Check sheet for the modelled part. Datum: model origin and axes. Units: mm. Face numbers are marked on the shaded views. Give positions to 0.01 mm unless a question says otherwise; leave off trailing zeros. Order: outer loops, then holes, each group sorted by start corner. A loop starts at its lowest first (then second) coordinate and runs counter-clockwise, first axis right, second up. Notation, with made-up numbers: (53, -22.75) -> (68, -22.75) arc R10 cw to (68, -13.75) -> close; hole circle Ø6 at (76, 40.25). An arc over 180 degrees is marked (long way). Write each question's results on one line, items separated by ' | '.
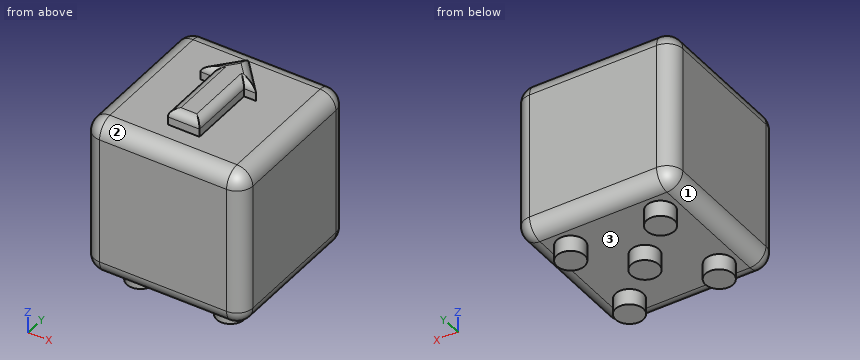
from build123d import *

# Parameters (mm, degrees)
F0_W     = 10
F0_H     = 10
F0_R     = 0.875
F1_DEPTH = 10
F2_DEPTH = 1
F3_R     = 1
F5_DEPTH = 1
F6_R     = 0.5


with BuildPart() as f1:
    # F0 (on Top) → F1 (new body)
    with BuildSketch(Plane.XY):
        Rectangle(F0_W, F0_H)
        with Locations((-2.828427, -2.828427)):
            Circle(F0_R, mode=Mode.SUBTRACT)
        with Locations((2.828427, -2.828427)):
            Circle(F0_R, mode=Mode.SUBTRACT)
        with Locations((-2.828427, 2.828427)):
            Circle(F0_R, mode=Mode.SUBTRACT)
        Circle(F0_R, mode=Mode.SUBTRACT)
        with Locations((2.828427, 2.828427)):
            Circle(F0_R, mode=Mode.SUBTRACT)
        with Locations((-2.828427, -2.828427)):
            Circle(F0_R)
        with Locations((-2.828427, 2.828427)):
            Circle(F0_R)
        with Locations((2.828427, 2.828427)):
            Circle(F0_R)
        with Locations((2.828427, -2.828427)):
            Circle(F0_R)
        Circle(F0_R)
    extrude(amount=F1_DEPTH)

    # F0 (on Top) → F2 (join)
    with BuildSketch(Plane.XY):
        with Locations((2.828427, 2.828427)):
            Circle(F0_R)
        with Locations((-2.828427, 2.828427)):
            Circle(F0_R)
        with Locations((-2.828427, -2.828427)):
            Circle(F0_R)
        with Locations((2.828427, -2.828427)):
            Circle(F0_R)
        Circle(F0_R)
    extrude(amount=-F2_DEPTH)

    # F3
    f3_edges = [f1.edges().sort_by_distance(p)[0] for p in [
        (5, 5, 5),
        (0, 5, 0),
        (5, 0, 0),
        (-5, 0, 0),
        (-5, 5, 5),
        (-5, -5, 5),
        (-5, 0, 10),
        (0, -5, 10),
        (5, 0, 10),
        (0, 5, 10),
        (5, -5, 5),
        (0, -5, 0),
    ]]
    fillet(f3_edges, radius=F3_R)

    # F4 (on face) → F5 (join)
    with BuildSketch(Plane.XY.offset(10)):
        Polygon((-1, 1.273247), (-1, 0), (-1, -3.015627), (1, -3.015627), (1, 1.273247), (1.75, 1.273247), (0, 3.273247), (-1.75, 1.273247), align=None)
    extrude(amount=F5_DEPTH)

    # F6
    f6_edges = [f1.edges().sort_by_distance(p)[0] for p in [
        (-0.875, 2.273247, 11),
        (-1.375, 1.273247, 11),
        (-1, -0.87119, 11),
        (0, -3.015627, 11),
        (1, -0.87119, 11),
        (1.375, 1.273247, 11),
        (0.875, 2.273247, 11),
    ]]
    fillet(f6_edges, radius=F6_R)


solid = f1.part
1. Section check C-C on x = 2.25. Record the cut outline in (y, z).
Verdict:
outline: (-5, 1) arc R1 ccw to (-4, 0) -> (-3.48, 0) -> (-3.48, -1) -> (-2.17, -1) -> (-2.17, 0) -> (2.17, 0) -> (2.17, -1) -> (3.48, -1) -> (3.48, 0) -> (4, 0) arc R1 ccw to (5, 1) -> (5, 9) arc R1 ccw to (4, 10) -> (-4, 10) arc R1 ccw to (-5, 9) -> close
2. Mould release check, pull along Y, two halves, no side actions. Record for the marked faces 1, 2 and 3: +Y half, -Y half, draft (parallel to the pull), parting line (faces both ways), or undercut.
Verdict:
face 1: draft | face 2: -Y half | face 3: undercut
3. Material ranges on probe 1 along Z at (x, y) = (-0.5, -1); probe 2 along Z at (x, y) = (-3, -0.25); probe 3 along Y at (x, z) = (2.25, -0.25), recorded low to high. Write a range as from..to.
Verdict:
probe 1: z = 0..11 | probe 2: z = 0..10 | probe 3: y = -3.48..-2.17, 2.17..3.48
4. Gauge pin test, flat ends, axial feed: pin 1 Ø0.6 at (y, z) = (-0.5, 10.5) entering from -X; pin 2 Ø0.6 at (y, z) = (-0.5, 10.5) entering from +X; pin 3 Ø0.6 at (x, z) = (0, 10) entering from -Y. Record the tip position at first contact, or that the pin passes through.
Verdict:
pin 1: stops at x = -1 | pin 2: stops at x = 1 | pin 3: stops at y = -4.71
5. Section check A-A on y = 0. Record the cut outline in (x, z) (3 decimals), then the cut area to 3 significant figures.
Verdict:
outline: (-5, 1) arc R1 ccw to (-4, 0) -> (-0.875, 0) -> (-0.875, -1) -> (0.875, -1) -> (0.875, 0) -> (4, 0) arc R1 ccw to (5, 1) -> (5, 9) arc R1 ccw to (4, 10) -> (1, 10) -> (1, 10.5) arc R0.5 ccw to (0.5, 11) -> (-0.5, 11) arc R0.5 ccw to (-1, 10.5) -> (-1, 10) -> (-4, 10) arc R1 ccw to (-5, 9) -> close | area: 103 mm^2
6. Section check D-D on y = -1.5. Record the cut outline in (x, z), then the cut area to 3 significant figures.
Verdict:
outline: (-5, 1) arc R1 ccw to (-4, 0) -> (4, 0) arc R1 ccw to (5, 1) -> (5, 9) arc R1 ccw to (4, 10) -> (1, 10) -> (1, 10.5) arc R0.5 ccw to (0.5, 11) -> (-0.5, 11) arc R0.5 ccw to (-1, 10.5) -> (-1, 10) -> (-4, 10) arc R1 ccw to (-5, 9) -> close | area: 101 mm^2
7. Section check B-B on z = 0.25. Record the cut outline in (x, y), then the cut area to 3 significant figures.
Verdict:
outline: (-4.66, -4) arc R0.66 ccw to (-4, -4.66) -> (4, -4.66) arc R0.66 ccw to (4.66, -4) -> (4.66, 4) arc R0.66 ccw to (4, 4.66) -> (-4, 4.66) arc R0.66 ccw to (-4.66, 4) -> close | area: 86.5 mm^2
